Autodesk Inventor part; units mm, degrees
ref_plane "YZ Plane" through (0, 0, 0) normal (1, 0, 0) x (0, 1, 0)
ref_plane "XZ Plane" through (0, 0, 0) normal (0, 1, 0) x (-1, 0, 0)
ref_plane "XY Plane" through (0, 0, 0) normal (0, 0, 1) x (1, 0, 0)
sketch "Sketch1" plane through (0, 0, 0) normal (0, 1, 0) x (-1, 0, 0)
  line L0 (0, 0) -> (65, 0)
  line L1 (65, 0) -> (65, -65)
  line L2 (65, -65) -> (0, -65)
  line L3 (0, -65) -> (0, 0)
  line L4 (0, 0) -> (-80, 0)
  line L5 (-80, 0) -> (-80, -65)
  line L6 (-80, -65) -> (0, -65)
  line L7 (0, -65) -> (0, 0)
  circle A0 centre (59.49, -9) radius 2.75
  circle A1 centre (59.49, -56) radius 2.75
  circle A2 centre (12.49, -9) radius 2.75
  circle A3 centre (12.49, -56) radius 2.75
  line L8 (-40, 0) -> (-40, -12.5)
  line L9 (-40, -12.5) -> (-40, -52.5)
  line L10 (-70, -12.5) -> (-10, -12.5) construction
  line L11 (-70, -15.25) -> (-10, -15.25)
  line L12 (-10, -9.75) -> (-70, -9.75)
  arc A4 (-70, -9.75) -> (-70, -15.25) centre (-70, -12.5) ccw
  arc A5 (-10, -15.25) -> (-10, -9.75) centre (-10, -12.5) ccw
  line L13 (-70, -52.5) -> (-10, -52.5) construction
  line L14 (-70, -55.25) -> (-10, -55.25)
  line L15 (-10, -49.75) -> (-70, -49.75)
  arc A6 (-70, -49.75) -> (-70, -55.25) centre (-70, -52.5) ccw
  arc A7 (-10, -55.25) -> (-10, -49.75) centre (-10, -52.5) ccw
  line L16 (-40, -52.5) -> (20, -52.5) construction
  circle A8 centre (32.5, -32.5) radius 22.5
  line L17 (32.5, -32.5) -> (48.4099, -16.5901)
  line L18 (32.5, -32.5) -> (55, -32.5) construction
  circle A9 centre (48.4099, -16.5901) radius 2.75
  circle A10 centre (16.5901, -16.5901) radius 2.75
  circle A11 centre (16.5901, -48.4099) radius 2.75
  circle A12 centre (48.4099, -48.4099) radius 2.75
  circle A13 centre (32.5, -32.5) radius 19.1
  dimension "d31" = 45
  dimension "d0" = 65
  dimension "d1" = 65
  dimension "d2" = 80
  dimension "d3" = 65
  dimension "d4" = 5.5
  dimension "d5" = 5.51
  dimension "d6" = 9
  dimension "d9" = 47
  dimension "d12" = 47
  dimension "d15" = 12.5
  dimension "d16" = 40
  dimension "d17" = 30
  dimension "d18" = 5.5
  dimension "d19" = 30
  dimension "d20" = 0
  dimension "d21" = 5.5
  dimension "d32" = 32.5
  dimension "d33" = 32.5
  dimension "d34" = 45
  dimension "d35" = 5.5
  dimension "d38" = 360
  dimension "d40" = 38.2
extrude "Extrusion3" add sketch "Sketch1" along normal blind 6 contours L0 L1 L2 L3 | L3 L6 L5 L4 | A8 A12 A11 A10 A9
fillet "Fillet3" radius 5 4 edges at (-65, 3, 0) (-65, 3, -65) (80, 3, -65) (80, 3, 0)
properties part number "NEMA23_FaceMount"
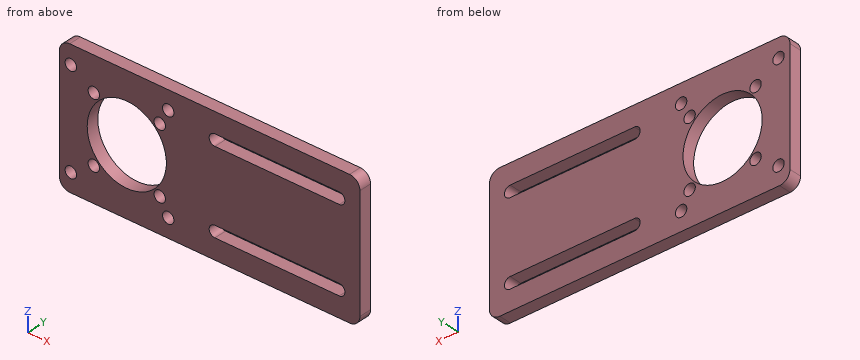
Design review of the part built by this model. Coordinates are the model's own, in mm. Coordinates: 2 decimals unless noted, no trailing zeros. Order: outer loops, then holes, each group sorted by start corner. A loop starts at its lowest first (then second) coordinate and runs counter-clockwise, first axis right, second up. Notation, with made-up numbers: (2.5, 53.5) -> (14.5, 53.5) arc R23 cw to (14.5, 74.5) -> close; hole circle Ø9 at (-31, 14.25). An arc over 180 degrees is marked (long way). One line per item, written item: value. Start each with the question number.
Q1. Take a section at C-C, the plane z = -37. State the section outline as (x, y) points.
Q2. Take a section at B-B, the plane x = -32.5. State the section outline as (y, z) points.
Q3. Insertion check: pin 1 Ø23 at (x, z) = (-32.5, -32.5) entering from +Y. The pin has a flat end and moves straight along its axis. Give the tip position at first contact, or say it passes through.
Q4. Take a section at D-D, the plane y = 2.55. Give the number of separate pieces and of enclosed holes in the cut face, then the cut area to 3 significant figures.
Q5. Take a section at A-A, the plane x = 42.5. State the section outline as (y, z) points.
Q6. For probe 1 along Z at (x, y) = (11, 2.75); probe 2 along X at (y, z) = (2.25, -32.5); probe 3 along X at (y, z) = (2.8, -48), list the stretches that pass through material, from the lowest coordinate up.
Values follow:
1. outline: (-65, 0) -> (-51.06, 0) -> (-51.06, 6) -> (-65, 6) -> close; (-13.94, 0) -> (80, 0) -> (80, 6) -> (-13.94, 6) -> close
2. outline: (0, -65) -> (6, -65) -> (6, -51.6) -> (0, -51.6) -> close; (0, -13.4) -> (6, -13.4) -> (6, 0) -> (0, 0) -> close
3. pin 1: passes through
4. separate pieces: 1
4. enclosed holes: 11
4. area: 7,360 mm2
5. outline: (0, -65) -> (6, -65) -> (6, -55.25) -> (0, -55.25) -> close; (0, -49.75) -> (6, -49.75) -> (6, -15.25) -> (0, -15.25) -> close; (0, -9.75) -> (6, -9.75) -> (6, 0) -> (0, 0) -> close
6. probe 1: z = -65 to -55.25, -49.75 to -15.25, -9.75 to 0
6. probe 2: x = -65 to -51.6, -13.4 to 80
6. probe 3: x = -65 to -51.13, -45.69 to -43.66, -21.34 to -19.31, -13.87 to 80
